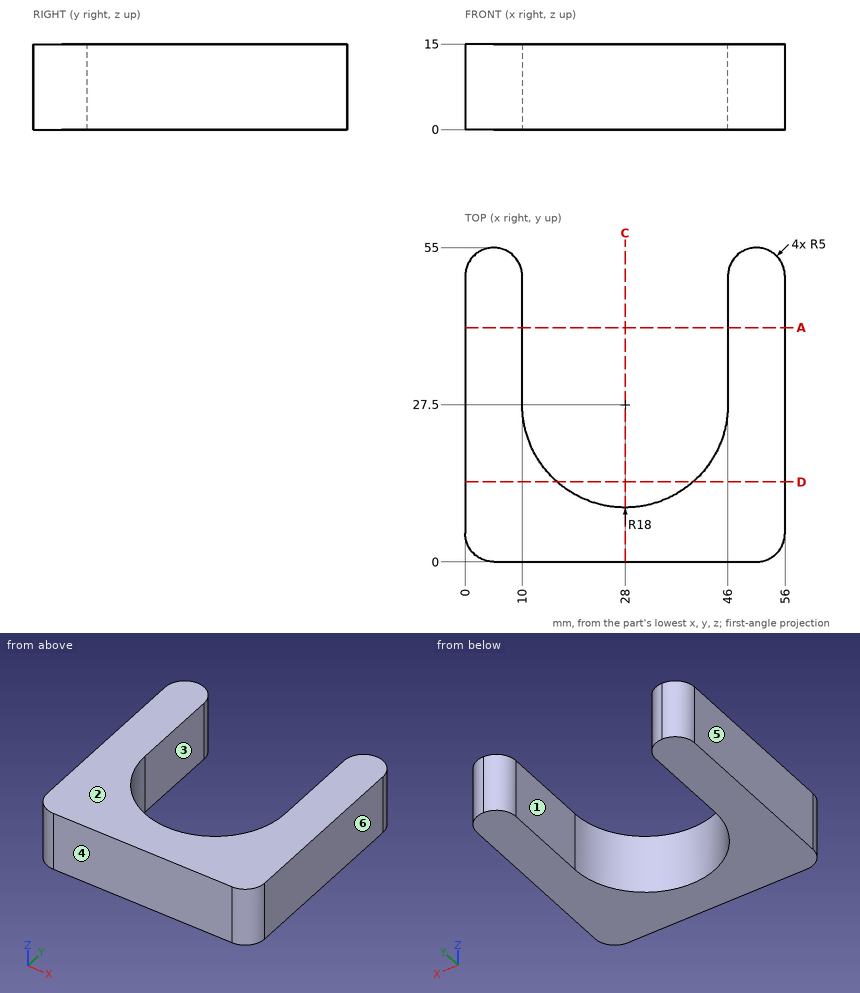
Here's the drawing with two shaded views (mm, measured from the low corner). I have some questions. A direction names the side the tool comes from. Coordinates: 2 decimals unless noted, no trailing zeros. Loops run counter-clockwise (first coordinate to the right, second up) from the corner with the lowest first, then second, coordinate; pieces in that order, holes last. Notation, with made-up numbers: M 41.5,82 L 79.5,82 A35 ccw 79.5,116 Z; hole C 29.25,-15.75 d8. An arc over 180 degrees is marked long. Answer as CSV lines item,"result". Start each with the question number.
1. Suppose I cut it at D-D, the plane y = 14. List the corners of the cut face in (x, z) for me, plus the area to 3 significant figures.
2. Suppose I cut it at C-C, the plane x = 28. List the corners of the cut face in (y, z) for me.
3. For pin 1 Ø3 at (x, z) = (10.5, 8.5) entering from -Y; pin 2 Ø5 at (x, z) = (15.5, 13) entering from +Y; pin 3 Ø3 at (x, z) = (40.5, 7.5) entering from +Y, each with a flat end and sliding along its axis, tell me the tip position at first contact or that it passes through.
4. For the marked faces 1 and 2, which set-ups out of +Z, -Z, +X, -X, +Y, -Y let a thin tool reach every point of the face, with its end or its side?
5. If I drill on probe 1 along X at (y, z) = (49.5, 13.25); probe 2 along X at (y, z) = (26, 4.5); probe 3 along Y at (x, z) = (2, 5.75), over which ranges is the centre line in solid material (lowest first)? Write a range as [from, to].
6. Thinking about a two-plate mould opening in X: for the marked faces 3, 4, 5 and 6, which applies, +X half, -X half, draft (parallel to the pull), parting line (faces both ways), or undercut?
7. Suppose I cut it at A-A, the plane y = 41. List the corners of the cut face in (x, z) for me.
Output:
1,outline,"M 0,0 L 16.09,0 L 16.09,15 L 0,15 Z; M 39.91,0 L 56,0 L 56,15 L 39.91,15 Z"
1,area,"483 mm^2"
2,outline,"M 0,0 L 9.5,0 L 9.5,15 L 0,15 Z"
3,pin 1,"stops at y = 0"
3,pin 2,"stops at y = 17.55"
3,pin 3,"stops at y = 16.19"
4,face 1,"+Z, -Z, +Y"
4,face 2,"+Z, +X, -X, +Y, -Y"
5,probe 1,"x = [0, 10], [46, 56]"
5,probe 2,"x = [0, 10.06], [45.94, 56]"
5,probe 3,"y = [1, 54]"
6,face 3,"undercut"
6,face 4,"draft"
6,face 5,"-X half"
6,face 6,"+X half"
7,outline,"M 0,0 L 10,0 L 10,15 L 0,15 Z; M 46,0 L 56,0 L 56,15 L 46,15 Z"
